Check sheet for the modelled part. Datum: model origin and axes. Units: mm. A direction names the side the tool comes from. Coordinates: 2 decimals unless noted, no trailing zeros. Write each question's results on one line, items separated by ' | '. Start each with the question number.
1. Thickness scan on line 1 (X direction, y = 1, z = 240.3); line 2 (X direction, y = -28, z = 241.9); line 3 (X direction, y = -25, z = 241.5). Record the ranges inside material, lowest first. Write a range as [from, to].
2. Gauge pin test, flat ends, axial feed: P1, Ø1, axis at x = 11.5, z = 243, coming from the -Y side; P2, Ø1, axis at x = 0.5, z = 242, coming from the -Y side; P3, Ø1.8, axis at x = 32.01, y = -5.36, coming from the +Z side. Record the tip position at first contact, or that the pin passes through.
3. Tool access check on faces 1 (the face through (33.68, 2.23, 241.57)), 2 (the face through (1.574, -29, 242)). Record the directions out of +Z, -Z, +X, -X, +Y, -Y that give a thin tool (end or side, any length) a straight path to the whole face; none if there is none.
4. Cross-section at A-A (z = 241.8). Give the number of separate pieces and of enclosed holes in the cut face, and give its area (3 significant figures).
5. Draft check along Y on faces 3 (the face through (-33.68, 2.3, 241.57)), 4 (the face through (0, -23.8, 242)), 5 (the face through (-32.215, -8.12, 241.61)). Enter one of: released by +Y, released by -Y, zero draft, split by the parting line, or undercut.
```python
from build123d import *

# Parameters (mm, degrees)
BOSS_EXTRUDE1_DEPTH = 3.175
SKETCH4_R           = 1
CUT_EXTRUDE2_DEPTH  = 3.175
SKETCH5_W           = 3.175
SKETCH5_H           = 10.970571453
CUT_EXTRUDE3_DEPTH  = 48.905713025


with BuildPart() as part:
    # Sketch1 → Boss-Extrude1 (new body)
    with BuildSketch(Plane.XY.offset(240)):
        with BuildLine():
            Line((-33.799525455, -0.017072147), (-33.740147252, -3.418847174))
            add(Edge.make_bspline(
                [(-33.740147252, -3.418847174), (-33.521913435, -5.496739744), (-33.121758608, -7.52360336), (-32.245655467, -10.48651683), (-31.738647045, -11.948631126), (-31.127755378, -13.381606109), (-30.697366268, -14.330435347), (-30.470378572, -14.801900059), (-29.290211733, -17.119612441), (-27.644930506, -19.740333777), (-25.646898465, -22.113857284), (-24.588376817, -23.258919171), (-24.224726915, -23.634521718), (-23.482012785, -24.367327148), (-21.59014774, -26.150424449), (-18.705670827, -28.317861845), (-15.980786711, -29.823605713), (-14.107006772, -30.74768667), (-13.152701084, -31.164175695), (-10.256242476, -32.27934775), (-7.777960893, -32.988270972), (-5.214339656, -33.405899808), (-4.181967985, -33.549320099), (-3.661328308, -33.60925586), (-2.104532681, -33.751997759), (-1.069213869, -33.798542764), (2.029597644, -33.801687472), (4.085962141, -33.622116253), (7.155117004, -33.058726493), (8.178081257, -32.820670852), (10.177000978, -32.256577633), (11.158104767, -31.929888742), (14.04936497, -30.823232748), (15.907936031, -29.917809181), (18.13673294, -28.556406158), (18.576889104, -28.273087614), (19.438710135, -27.689460729), (20.706973253, -26.786573761), (21.903631517, -25.803366446), (23.438553372, -24.424422105), (24.544411843, -23.339363165), (25.578640539, -22.173955923), (26.251776296, -21.378677652), (26.580969723, -20.970778515), (28.17094662, -18.902925334), (29.269671397, -17.152899222), (30.678907287, -14.395868232), (31.108821176, -13.454846631), (31.884053374, -11.526054988), (32.230015293, -10.534907216), (33.119638114, -7.539302803), (33.521651228, -5.499562958), (33.740182048, -3.418847117)],
                knots=[0, 0, 0, 0, 0.0625, 0.0625, 0.09375, 0.109375, 0.109375, 0.125, 0.125, 0.1875, 0.21875, 0.21875, 0.234375, 0.234375, 0.25, 0.3125, 0.34375, 0.34375, 0.375, 0.375, 0.4375, 0.453125, 0.453125, 0.46875, 0.46875, 0.5, 0.5, 0.5625, 0.5625, 0.59375, 0.59375, 0.625, 0.625, 0.6875, 0.6875, 0.703125, 0.703125, 0.71875, 0.75, 0.75, 0.78125, 0.796875, 0.796875, 0.8125, 0.8125, 0.875, 0.875, 0.90625, 0.90625, 0.9375, 0.9375, 1, 1, 1, 1], degree=3))
            Line((33.740182048, -3.418847117), (33.799560251, -0.017072147))
            Line((33.799560251, -0.017072147), (33.560412457, 4.546139609))
            add(Edge.make_bspline(
                [(33.560412457, 4.546139609), (33.282065399, 6.567374379), (32.831372803, 8.534230691), (31.894626922, 11.402256897), (31.361087401, 12.815708643), (30.729491779, 14.19822173), (30.286610148, 15.113013144), (30.053701075, 15.567925007), (28.845742701, 17.805295292), (27.73617385, 19.487837269), (25.852855801, 21.84749908), (25.188593752, 22.606698061), (23.786460552, 24.069913543), (23.045059446, 24.776640829), (20.752328135, 26.778284029), (18.311067746, 28.558159122), (15.640647898, 29.995877244), (14.266739996, 30.656956524), (13.801141084, 30.868163008), (12.864758887, 31.267971853), (12.393699461, 31.456783193), (10.024605965, 32.347483289), (7.115279765, 33.1594713), (4.10232218, 33.57067126), (2.070213322, 33.754033964), (1.053662161, 33.799146951), (-1.978663229, 33.802802386), (-4.487220386, 33.587681269), (-6.97150073, 33.084409187), (-7.963243622, 32.859726611), (-8.459399615, 32.73533069), (-9.933669217, 32.329805435), (-10.897365307, 32.016750487), (-13.734609646, 30.957514861), (-15.554750033, 30.092235814), (-17.734673571, 28.798227251), (-18.165893543, 28.52880028), (-19.018645374, 27.968342063), (-19.439187613, 27.677889019), (-20.673952363, 26.783179445), (-21.465207676, 26.153069384), (-23.74871726, 24.167631397), (-25.151109466, 22.717611147), (-26.742507526, 20.734807748), (-27.053436756, 20.328702835), (-27.654958645, 19.504501759), (-28.525682186, 18.252011757), (-29.304349299, 16.952301265), (-30.745483656, 14.293275375), (-31.551336523, 12.44113352), (-32.506911863, 9.533039369), (-32.781055324, 8.547728647), (-33.237634192, 6.561909519), (-33.420905282, 5.558925362), (-33.560377664, 4.546139552)],
                knots=[0, 0, 0, 0, 0.0625, 0.0625, 0.09375, 0.109375, 0.109375, 0.125, 0.125, 0.1875, 0.1875, 0.21875, 0.21875, 0.25, 0.25, 0.3125, 0.34375, 0.34375, 0.359375, 0.359375, 0.375, 0.375, 0.4375, 0.46875, 0.46875, 0.5, 0.5, 0.5625, 0.578125, 0.578125, 0.59375, 0.59375, 0.625, 0.625, 0.6875, 0.6875, 0.703125, 0.703125, 0.71875, 0.71875, 0.75, 0.75, 0.8125, 0.8125, 0.828125, 0.828125, 0.84375, 0.875, 0.875, 0.9375, 0.9375, 0.96875, 0.96875, 1, 1, 1, 1], degree=3))
            Line((-33.560377664, 4.546139552), (-33.799525455, -0.017072147))
        make_face()
    extrude(amount=BOSS_EXTRUDE1_DEPTH)

    # Sketch4 → Cut-Extrude2 (cut)
    with BuildSketch(Plane.XY.offset(243.175)):
        with Locations((32.009302375, -5.358989516)):
            Circle(SKETCH4_R)
        with Locations((-31.216064399, -8.164436653)):
            Circle(SKETCH4_R)
    extrude(amount=-CUT_EXTRUDE2_DEPTH, mode=Mode.SUBTRACT)

    # Sketch5 → Cut-Extrude3 (cut, through all)
    with BuildSketch(Plane.XY.offset(243.175)):
        with Locations((-0.013127042, -29.284890239)):
            Rectangle(SKETCH5_W, SKETCH5_H)
    extrude(amount=-CUT_EXTRUDE3_DEPTH, mode=Mode.SUBTRACT)


solid = part.part
```
Established:
1) line 1: [-33.75, 33.75] | line 2: [-18.98, -1.6], [1.57, 18.98] | line 3: [-22.8, -1.6], [1.57, 22.8]
2) P1: y = -31.97 | P2: y = -23.8 | P3: through
3) face 1: +Z, -Z, +X, +Y | face 2: +Z, -Z, -Y
4) separate pieces: 1 | enclosed holes: 2 | area: 3,560 mm^2
5) face 3: released by +Y | face 4: released by -Y | face 5: undercut
